Design review of the part built by this model. Coordinates are the model's own, in mm. A direction names the side the tool comes from. Give positions to 0.01 mm unless a question says otherwise; leave off trailing zeros. Order: outer loops, then holes, each group sorted by start corner. A loop starts at its lowest first (then second) coordinate and runs counter-clockwise, first axis right, second up. Notation, with made-up numbers: (70.25, 80.5) -> (92.25, 80.5) arc R21 ccw to (92.25, 93.5) -> close; hole circle Ø5 at (53, -13). An arc over 180 degrees is marked (long way). Return JSON: item names as keys, results as strings.
```python
from build123d import *

# Parameters (mm, degrees)
SKETCH1_W           = 70
SKETCH1_H           = 119
BOSS_EXTRUDE1_DEPTH = 35
SKETCH2_R           = 8
CUT_EXTRUDE1_DEPTH  = 8
CUT_EXTRUDE2_DEPTH  = 32
SKETCH4_R           = 7.5
CUT_EXTRUDE3_DEPTH  = 8
SKETCH5_W           = 16
SKETCH5_H           = 20
SKETCH5_W_2         = 23
CUT_EXTRUDE4_DEPTH  = 78.396705356
CUT_EXTRUDE5_DEPTH  = 5
SKETCH7_W           = 18
SKETCH7_H           = 32
CUT_EXTRUDE6_DEPTH  = 2
SKETCH8_W           = 32
SKETCH8_H           = 22
CUT_EXTRUDE7_DEPTH  = 2
SKETCH9_W           = 22
SKETCH9_H           = 32
CUT_EXTRUDE8_DEPTH  = 2
SKETCH10_W          = 32
SKETCH10_H          = 18
CUT_EXTRUDE9_DEPTH  = 2
CUT_EXTRUDE11_DEPTH = 5
SKETCH13_W          = 20
SKETCH13_H          = 32
CUT_EXTRUDE12_DEPTH = 2
SKETCH14_W          = 22
SKETCH14_H          = 32
CUT_EXTRUDE13_DEPTH = 2
SKETCH15_W          = 32
SKETCH15_H          = 18
CUT_EXTRUDE14_DEPTH = 2
SKETCH16_W          = 18
SKETCH16_H          = 32
CUT_EXTRUDE15_DEPTH = 2
SKETCH17_W          = 32
SKETCH17_H          = 20.10525169
CUT_EXTRUDE16_DEPTH = 2
FILLET1_R           = 5
FILLET3_R           = 5
FILLET4_R           = 5
SKETCH18_R          = 1.5
CUT_EXTRUDE17_DEPTH = 10
SKETCH19_R          = 0.9
CUT_EXTRUDE18_DEPTH = 10
BOSS_EXTRUDE3_DEPTH = 6
BOSS_EXTRUDE4_START = -6
BOSS_EXTRUDE4_DEPTH = 6


with BuildPart() as part:
    # Sketch1 → Boss-Extrude1 (new body)
    with BuildSketch(Plane.XY):
        Rectangle(SKETCH1_W, SKETCH1_H)
    extrude(amount=BOSS_EXTRUDE1_DEPTH)

    # Sketch2 → Cut-Extrude1 (cut)
    with BuildSketch(Plane.ZY.offset(35)):
        with Locations((35, -19.5)):
            Circle(SKETCH2_R)
    extrude(amount=-CUT_EXTRUDE1_DEPTH, mode=Mode.SUBTRACT)

    # Sketch3 → Cut-Extrude2 (cut)
    with BuildSketch(Plane.XY.offset(35)):
        Polygon((-27, 54.5), (-13, 54.5), (-13, 27), (-7, 27), (-7, 34.5), (7, 34.5), (7, -12), (13, -12), (13, 54.5), (27, 54.5), (27, -34.5), (13, -34.5), (13, -27), (7, -27), (7, -54.5), (-7, -54.5), (-7, 12), (-13, 12), (-13, -34.5), (-27, -34.5), align=None)
    extrude(amount=-CUT_EXTRUDE2_DEPTH, mode=Mode.SUBTRACT)

    # Sketch4 → Cut-Extrude3 (cut)
    with BuildSketch(Plane(origin=(35, 0, 0), x_dir=(0, 0, -1), z_dir=(1, 0, 0))):
        with Locations((-35, 19.5)):
            Circle(SKETCH4_R)
    extrude(amount=-CUT_EXTRUDE3_DEPTH, mode=Mode.SUBTRACT)

    # Sketch5 → Cut-Extrude4 (cut, through all)
    with BuildSketch(Plane.XY.offset(35)):
        with Locations((0, 49.5)):
            Rectangle(SKETCH5_W, SKETCH5_H)
        with Locations((23.5, -49.5)):
            Rectangle(SKETCH5_W_2, SKETCH5_H)
        with Locations((-23.5, -49.5)):
            Rectangle(SKETCH5_W_2, SKETCH5_H)
    extrude(amount=-CUT_EXTRUDE4_DEPTH, mode=Mode.SUBTRACT)

    # Sketch6 → Cut-Extrude5 (cut)
    with BuildSketch(Plane(origin=(35, 0, 0), x_dir=(0, 0, -1), z_dir=(1, 0, 0))):
        with BuildLine():
            Line((-32, 59.5), (0, 59.5))
            Line((0, 59.5), (0, -39.5))
            Line((0, -39.5), (-32, -39.5))
            Line((-32, -39.5), (-32, 9.437694101))
            ThreePointArc((-32, 9.437694101), (-24.5, 19.5), (-32, 29.562305899))
            Line((-32, 29.562305899), (-32, 59.5))
        make_face()
    extrude(amount=-CUT_EXTRUDE5_DEPTH, mode=Mode.SUBTRACT)

    # Sketch7 → Cut-Extrude6 (cut)
    with BuildSketch(Plane.XZ.offset(39.5)):
        with Locations((21, 16)):
            Rectangle(SKETCH7_W, SKETCH7_H)
    extrude(amount=-CUT_EXTRUDE6_DEPTH, mode=Mode.SUBTRACT)

    # Sketch8 → Cut-Extrude7 (cut)
    with BuildSketch(Plane(origin=(12, 0, 0), x_dir=(0, 0, -1), z_dir=(1, 0, 0))):
        with Locations((-16, -48.5)):
            Rectangle(SKETCH8_W, SKETCH8_H)
    extrude(amount=-CUT_EXTRUDE7_DEPTH, mode=Mode.SUBTRACT)

    # Sketch9 → Cut-Extrude8 (cut)
    with BuildSketch(Plane.XZ.offset(59.5)):
        with Locations((-1, 16)):
            Rectangle(SKETCH9_W, SKETCH9_H)
    extrude(amount=-CUT_EXTRUDE8_DEPTH, mode=Mode.SUBTRACT)

    # Sketch10 → Cut-Extrude9 (cut)
    with BuildSketch(Plane.ZY.offset(12)):
        with Locations((16, -48.5)):
            Rectangle(SKETCH10_W, SKETCH10_H)
    extrude(amount=-CUT_EXTRUDE9_DEPTH, mode=Mode.SUBTRACT)

    # Sketch12 → Cut-Extrude11 (cut)
    with BuildSketch(Plane.ZY.offset(35)):
        with BuildLine():
            Line((32, 59.5), (0, 59.5))
            Line((0, 59.5), (0, -39.5))
            Line((0, -39.5), (32, -39.5))
            Line((32, -39.5), (32, -30.083005244))
            ThreePointArc((32, -30.083005244), (24, -19.5), (32, -8.916994756))
            Line((32, -8.916994756), (32, 59.5))
        make_face()
    extrude(amount=-CUT_EXTRUDE11_DEPTH, mode=Mode.SUBTRACT)

    # Sketch13 → Cut-Extrude12 (cut)
    with BuildSketch(Plane.XZ.offset(39.5)):
        with Locations((-20, 16)):
            Rectangle(SKETCH13_W, SKETCH13_H)
    extrude(amount=-CUT_EXTRUDE12_DEPTH, mode=Mode.SUBTRACT)

    # Sketch14 → Cut-Extrude13 (cut)
    with BuildSketch(Plane(origin=(0, 59.5, 0), x_dir=(1, 0, 0), z_dir=(0, 1, 0))):
        with Locations((19, -16)):
            Rectangle(SKETCH14_W, SKETCH14_H)
        with Locations((-19, -16)):
            Rectangle(SKETCH14_W, SKETCH14_H)
    extrude(amount=-CUT_EXTRUDE13_DEPTH, mode=Mode.SUBTRACT)

    # Sketch15 → Cut-Extrude14 (cut)
    with BuildSketch(Plane.ZY.offset(-8)):
        with Locations((16, 48.5)):
            Rectangle(SKETCH15_W, SKETCH15_H)
    extrude(amount=-CUT_EXTRUDE14_DEPTH, mode=Mode.SUBTRACT)

    # Sketch16 → Cut-Extrude15 (cut)
    with BuildSketch(Plane(origin=(0, 39.5, 0), x_dir=(1, 0, 0), z_dir=(0, 1, 0))):
        with Locations((1, -16)):
            Rectangle(SKETCH16_W, SKETCH16_H)
    extrude(amount=-CUT_EXTRUDE15_DEPTH, mode=Mode.SUBTRACT)

    # Sketch17 → Cut-Extrude16 (cut)
    with BuildSketch(Plane(origin=(-8, 0, 0), x_dir=(0, 0, -1), z_dir=(1, 0, 0))):
        with Locations((-16, 47.447374155)):
            Rectangle(SKETCH17_W, SKETCH17_H)
    extrude(amount=-CUT_EXTRUDE16_DEPTH, mode=Mode.SUBTRACT)

    # Fillet1
    fillet1_edges = [part.edges().sort_by_distance(p)[0] for p in [
        (-27, -34.5, 19),
        (-27, 54.5, 19),
        (-13, 54.5, 19),
        (-7, 34.5, 19),
        (7, 34.5, 19),
        (13, 54.5, 19),
        (27, 54.5, 19),
        (27, -34.5, 19),
        (13, -34.5, 19),
        (7, -54.5, 19),
        (-7, -54.5, 19),
        (-13, -34.5, 19),
    ]]
    fillet(fillet1_edges, radius=FILLET1_R)

    # Fillet3
    # the kernel refuses this fillet: 5 mm, written as the material it adds along each edge
    with BuildSketch(Plane(origin=(-10, -37.5, 0), x_dir=(0, -1, 0), z_dir=(0, 0, 1))) as fillet3_piece_1:
        with BuildLine():
            CenterArc((FILLET3_R, -FILLET3_R), FILLET3_R, 90, 90)
            Line((0, -FILLET3_R), (0, 0))
            Line((0, 0), (FILLET3_R, 0))
        make_face()
    extrude(amount=32)
    with BuildSketch(Plane(origin=(10, -37.5, 32), x_dir=(1, 0, 0), z_dir=(0, 0, -1)), Plane(origin=(10, 37.5, 0), x_dir=(0, 1, 0), z_dir=(0, 0, 1))) as fillet3_piece_2:
        with BuildLine():
            CenterArc((FILLET3_R, FILLET3_R), FILLET3_R, 180, 90)
            Line((0, FILLET3_R), (0, 0))
            Line((0, 0), (FILLET3_R, 0))
        make_face()
    extrude(amount=32)
    with BuildSketch(Plane(origin=(-10, 37.39474831, 32), x_dir=(1, 0, 0), z_dir=(0, 0, -1))) as fillet3_piece_3:
        with BuildLine():
            CenterArc((5, -4), FILLET3_R, 126.869897646, 53.130102354)
            Line((0, -4), (0, 0))
            Line((0, 0), (2, 0))
        make_face()
    extrude(amount=32)
    # the kernel refuses this fillet: 5 mm, written as the material it takes off along each edge
    with BuildSketch(Plane(origin=(-10, 57.5, -12.5), x_dir=(-1, 0, 0), z_dir=(0, 0, 1)), Plane(origin=(-30, -37.5, 32), x_dir=(0, 1, 0), z_dir=(0, 0, -1)), Plane(origin=(-10, -57.5, 32), x_dir=(0, 1, 0), z_dir=(0, 0, -1))) as fillet3_2_piece_1:
        with BuildLine():
            CenterArc((FILLET3_R, FILLET3_R), FILLET3_R, 180, 90)
            Line((0, FILLET3_R), (0, 0))
            Line((0, 0), (FILLET3_R, 0))
        make_face()
    extrude(amount=44.5, mode=Mode.SUBTRACT)
    with BuildSketch(Plane(origin=(-30, 57.5, 32), x_dir=(0, -1, 0), z_dir=(0, 0, -1)), Plane(origin=(30, -37.5, -12.5), x_dir=(-1, 0, 0), z_dir=(0, 0, 1)), Plane(origin=(30, 57.5, -12.5), x_dir=(0, -1, 0), z_dir=(0, 0, 1)), Plane(origin=(10, 57.5, 32), x_dir=(0, -1, 0), z_dir=(0, 0, -1)), Plane(origin=(10, -57.5, -12.5), x_dir=(-1, 0, 0), z_dir=(0, 0, 1))) as fillet3_2_piece_2:
        with BuildLine():
            CenterArc((FILLET3_R, -FILLET3_R), FILLET3_R, 90, 90)
            Line((0, -FILLET3_R), (0, 0))
            Line((0, 0), (FILLET3_R, 0))
        make_face()
    extrude(amount=44.5, mode=Mode.SUBTRACT)

    # Fillet4
    fillet4_edges = [part.edges().sort_by_distance(p)[0] for p in [
        (35, -39.5, 33.5),
        (12, -39.5, 33.5),
        (12, -59.5, 33.5),
        (-12, -59.5, 33.5),
        (-12, -39.5, 33.5),
        (-35, -39.5, 33.5),
        (8, 59.5, 33.5),
        (-8, 59.5, 33.5),
        (8, 39.5, 33.5),
        (-8, 39.5, 33.5),
        (-35, 59.5, 33.5),
        (35, 59.5, 33.5),
    ]]
    fillet(fillet4_edges, radius=FILLET4_R)

    # Sketch18 → Cut-Extrude17 (cut)
    with BuildSketch(Plane.XY.offset(35)):
        with Locations((-32, 56.5)):
            Circle(SKETCH18_R)
        with Locations((32, 56.5)):
            Circle(SKETCH18_R)
        with Locations((-32, -36.5)):
            Circle(SKETCH18_R)
        with Locations((-10, -36.5)):
            Circle(SKETCH18_R)
        with Locations((10, -36.5)):
            Circle(SKETCH18_R)
        with Locations((32, -36.5)):
            Circle(SKETCH18_R)
    extrude(amount=-CUT_EXTRUDE17_DEPTH, mode=Mode.SUBTRACT)

    # Sketch19 → Cut-Extrude18 (cut)
    with BuildSketch(Plane.XY.offset(35)):
        with Locations((-10, 56.5)):
            Circle(SKETCH19_R)
        with Locations((10, 56.5)):
            Circle(SKETCH19_R)
        with Locations((-10, -57)):
            Circle(SKETCH19_R)
        with Locations((10, -57)):
            Circle(SKETCH19_R)
    extrude(amount=-CUT_EXTRUDE18_DEPTH, mode=Mode.SUBTRACT)

    # Sketch20 → Boss-Extrude3 (add)
    with BuildSketch(Plane(origin=(13, 0, 0), x_dir=(0, 0, -1), z_dir=(1, 0, 0))):
        with BuildLine():
            Line((-35, -12), (-3, -12))
            Line((-3, -12), (-3, -27))
            Line((-3, -27), (-35, -27))
            ThreePointArc((-35, -27), (-27.5, -19.5), (-35, -12))
        make_face()
    extrude(amount=-BOSS_EXTRUDE3_DEPTH)

    # Sketch21 → Boss-Extrude4 (add)
    with BuildSketch(Plane.ZY.offset(13).offset(BOSS_EXTRUDE4_START)):
        with BuildLine():
            Line((35, 27), (3, 27))
            Line((3, 27), (3, 12))
            Line((3, 12), (35, 12))
            ThreePointArc((35, 12), (27.5, 19.5), (35, 27))
        make_face()
    extrude(amount=BOSS_EXTRUDE4_DEPTH)


solid = part.part
```
Item 1: For pin 1 (6 mm diameter, centred on x = -21, z = 14, fed in from -Y); pin 2 (6 mm diameter, centred on y = -35, z = 13.5, fed in from +X); pin 3 (5 mm diameter, centred on y = 32, z = 10.5, fed in from -X), all flat-tipped, find the tip position at first contact; note any pin that passes through.
Result set:
{"pin 1": "stops at y = -37.5", "pin 2": "stops at x = 30", "pin 3": "stops at x = -30"}
Item 2: Machinability: for faces 1 (the face through (-20, -37.5, 16)), 2 (the face through (-9.43, 58, 33.48)), 3 (the face through (20, 11, 3)), 4 (the face through (10, -47, 16)), which of the approach directions +Z, -Z, +X, -X, +Y, -Y give a long, thin tool a straight path to every point of the face, cutting with its end or side? Answer none if there is none.
Result set:
{"face 1": "-Z, -X, -Y", "face 2": "+Z, -Z, +Y", "face 3": "+Z", "face 4": "-Z, +X, -Y"}
Item 3: Add section B-B (x = -32). Give the boundary of the cut face in (y, z), plus the area to 3 significant figures.
Result set:
{"outline": "(-39.08, 32) -> (-38, 32) -> (-38, 35) -> (-39.08, 35) -> close; (-35, 32) -> (-30.08, 32) arc R11 ccw to (-8.92, 32) -> (55, 32) -> (55, 35) -> (-11.5, 35) arc R8 cw to (-27.5, 35) -> (-35, 35) -> close; (58, 32) -> (59.08, 32) -> (59.08, 35) -> (58, 35) -> close", "area": "301 mm^2"}
Item 4: Add section A-A (y = -19.5). Give the boundary of the cut face in (x, z).
Result set:
{"outline": "(-35, 24) -> (-30, 24) -> (-30, 0) -> (30, 0) -> (30, 32) -> (35, 32) -> (35, 35) -> (27, 35) -> (27, 3) -> (13, 3) -> (13, 27.5) -> (7, 27.5) -> (7, 3) -> (-7, 3) -> (-7, 35) -> (-13, 35) -> (-13, 3) -> (-27, 3) -> (-27, 27) -> (-35, 27) -> close"}
Item 5: Mouldability with a two-part tool opening along X and no side actions: class faces 5 (the face through (-32.5, -19.7, 24)), 6 (the face through (10.04, -19.66, 27.5)), 7 (the face through (-12, -50, 34)), 8 (the face through (-25.5, -33.07, 18.78)) as released by +X, released by -X, zero draft, split by the parting line, or undercut.
Result set:
{"face 5": "zero draft", "face 6": "undercut", "face 7": "released by -X", "face 8": "undercut"}
Item 6: Add section D-D (z = 9). Give the number of separate pieces and of enclosed holes in the cut face, plus the area to 3 significant figures.
Result set:
{"separate pieces": "1", "enclosed holes": "3", "area": "2,000 mm^2"}
Item 7: Wall thickness on L1, parallel to X at y = -7, z = 26.5; L2, parallel to X at y = 44, z = 13; L3, parallel to Y at x = -32, z = 33.35: over which ranges is each line inside the solid? List them lowest first. Write a range as [from, to].
Result set:
{"L1": "x = [-30, -27], [-13, -7], [7, 13], [27, 30]", "L2": "x = [-30, -27], [-13, -10], [10, 13], [27, 30]", "L3": "y = [-39.08, -38], [-35, -27.33], [-11.67, 55], [58, 59.08]"}
Item 8: Add section C-C (x = 20). Give the boundary of the cut face in (y, z).
Result set:
{"outline": "(-39.5, 32) -> (-37.5, 32) -> (-37.5, 0) -> (57.5, 0) -> (57.5, 32) -> (59.5, 32) -> (59.5, 35) -> (54.5, 35) -> (54.5, 3) -> (-34.5, 3) -> (-34.5, 35) -> (-39.5, 35) -> close"}
